Could you check a few things on this model? Use its own coordinates, in mm. Coordinates: 2 decimals unless noted, no trailing zeros. Write each loop counter-clockwise with the first axis right and the second up, starting at its lowest first coordinate (ties: lowest second). Pieces come first, ordered by that corner, then holes.
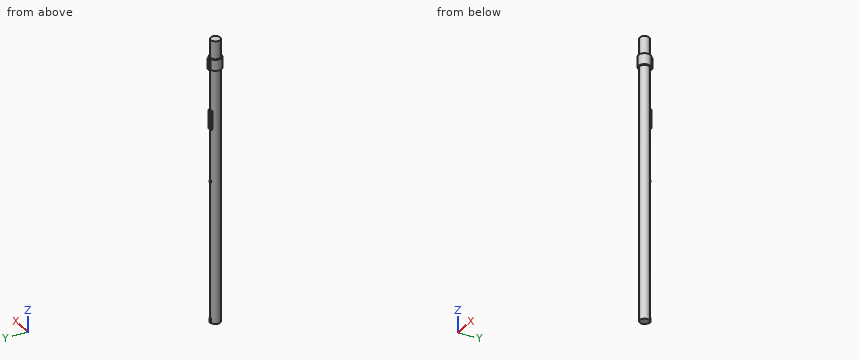
```python
from build123d import *

# Parameters (mm, degrees)
SKETCH1_R                = 17.5
BOSS_EXTRUDE1_DEPTH      = 1050
BOSS_EXTRUDE2_DEPTH      = 5
BOSS_EXTRUDE2_DEPTH_BACK = 5
SKETCH2_W                = 5
SKETCH2_H                = 5
BOSS_EXTRUDE3_START      = -40.50047623
SKETCH5_R                = 17.5
SKETCH5_R_2              = 11.1125
BOSS_EXTRUDE3_DEPTH      = 40.50047623
SKETCH7_R                = 22.225
BOSS_EXTRUDE4_DEPTH      = 40.50047623
SKETCH11_W               = 9.53
SKETCH11_H               = 8.74
BOSS_EXTRUDE5_DEPTH      = 40.50047623
SKETCH12_W               = 5
SKETCH12_H               = 5
BOSS_EXTRUDE6_DEPTH      = 18
SKETCH13_R               = 2
CUT_EXTRUDE1_DEPTH       = 10
SKETCH15_R               = 1
CUT_EXTRUDE3_DEPTH       = 10
SKETCH16_W               = 14
SKETCH16_H               = 10
BOSS_EXTRUDE7_DEPTH      = 70


with BuildPart() as part:
    # Sketch1 → Boss-Extrude1 (new body)
    with BuildSketch(Plane.XY):
        Circle(SKETCH1_R)
    extrude(amount=BOSS_EXTRUDE1_DEPTH)

    # Sketch2 → Boss-Extrude2 (add, two sides: drawn at the far end of the back side and taken through both)
    with BuildSketch(Plane.XY.offset(525).offset(-BOSS_EXTRUDE2_DEPTH_BACK)):
        with Locations((0, 17.5)):
            Rectangle(SKETCH2_W, SKETCH2_H)
    extrude(amount=BOSS_EXTRUDE2_DEPTH + BOSS_EXTRUDE2_DEPTH_BACK)

    # Sketch5 → Boss-Extrude3 (add)
    with BuildSketch(Plane.XY.offset(1050).offset(BOSS_EXTRUDE3_START)):
        Circle(SKETCH5_R)
        Circle(SKETCH5_R_2, mode=Mode.SUBTRACT)
    extrude(amount=BOSS_EXTRUDE3_DEPTH)

    # Sketch7 → Boss-Extrude4 (add)
    with BuildSketch(Plane.XY.offset(943)):
        Circle(SKETCH7_R)
    extrude(amount=BOSS_EXTRUDE4_DEPTH)

    # Sketch11 → Boss-Extrude5 (add)
    with BuildSketch(Plane.XY.offset(983.50047623)):
        with Locations((0, 22.225)):
            Rectangle(SKETCH11_W, SKETCH11_H)
    extrude(amount=-BOSS_EXTRUDE5_DEPTH)

    # Sketch12 → Boss-Extrude6 (add)
    with BuildSketch(Plane(origin=(0, 0, 0), x_dir=(-1, 0, 0), z_dir=(0, 0, -1))):
        with Locations((0, 17.5)):
            Rectangle(SKETCH12_W, SKETCH12_H)
    extrude(amount=-BOSS_EXTRUDE6_DEPTH)

    # Sketch13 → Cut-Extrude1 (cut)
    with BuildSketch(Plane(origin=(0, 20, 0), x_dir=(1, 0, 0), z_dir=(0, 1, 0))):
        with Locations(Location((0, -5, 0), (0, 0, 270))):
            Circle(SKETCH13_R)
    extrude(amount=-CUT_EXTRUDE1_DEPTH, mode=Mode.SUBTRACT)

    # Sketch15 → Cut-Extrude3 (cut)
    with BuildSketch(Plane(origin=(0, 20, 0), x_dir=(1, 0, 0), z_dir=(0, 1, 0))):
        with Locations(Location((0, -528.5, 0), (0, 0, 270))):
            Circle(SKETCH15_R)
    extrude(amount=-CUT_EXTRUDE3_DEPTH, mode=Mode.SUBTRACT)

    # Sketch16 → Boss-Extrude7 (add)
    with BuildSketch(Plane.XY.offset(790)):
        with Locations((0, 17.5)):
            Rectangle(SKETCH16_W, SKETCH16_H)
    extrude(amount=-BOSS_EXTRUDE7_DEPTH)


solid = part.part
```
1. I want a section at B-B on z = 814. Please give me the cut outline in (x, y), plus the area to 3 significant figures.
Verdict:
outline: circle Ø35 at (0, 0)
area: 962 mm2
2. Please list where these lines run through material, in increasing order: line 1 along X through (y, z) = (1, 284); line 2 along X through (y, z) = (15.25, 528.5); line 3 along X through (y, z) = (17.5, 528.5).
Verdict:
line 1: x = -17.47 to 17.47
line 2: x = -8.58 to -1, 1 to 8.58
line 3: x = -2.5 to -1, 1 to 2.5
3. For pin 1 (2 mm diameter, centred on y = 19, z = 527.5, fed in from +X); pin 2 (5.5 mm diameter, centred on x = -0.5, z = 8.5, fed in from +Y); pin 3 (3 mm diameter, centred on x = 16, z = 608, fed in from -Y), each with a flat end and sliding along its axis, tell me the tip position at first contact or that it passes through.
Verdict:
pin 1: stops at x = 2.5
pin 2: stops at y = 20
pin 3: stops at y = -9.8
4. I want a section at A-A on y = 0. Please give me the cut outline in (x, z) (3 decimals).
Verdict:
outline: (-22.225, 943) - (-17.5, 943) - (-17.5, 0) - (17.5, 0) - (17.5, 943) - (22.225, 943) - (22.225, 983.5) - (17.5, 983.5) - (17.5, 1050) - (-17.5, 1050) - (-17.5, 983.5) - (-22.225, 983.5) - close
